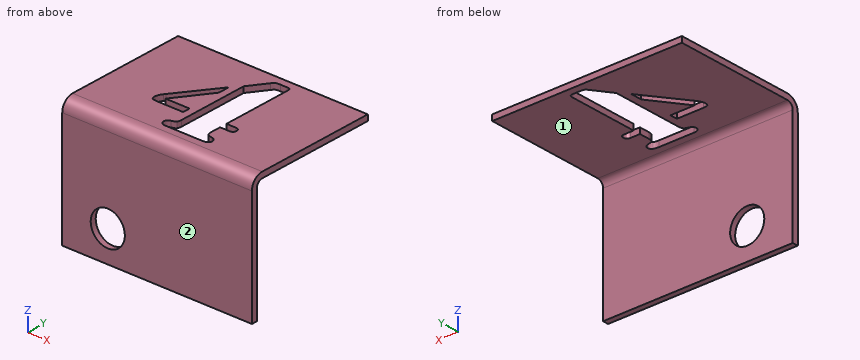
```python
from build123d import *

# Parameters (mm, degrees)
SKETCH1_W            = 50
SKETCH1_H            = 30
BASE_FLANGE1_DEPTH   = 1.51892
EDGE_FLANGE1_DEPTH   = 50
M8_CLEARANCE_HOLE1_D = 9
CUT_EXTRUDE1_DEPTH   = 55.277389816


# Sheet-metal steps are written as plain solids
with BuildPart() as part:
    # Sketch1 → Base-Flange1 (new body)
    with BuildSketch(Plane(origin=(0, 0, 0), x_dir=(1, 0, 0), z_dir=(0, 1, 0))):
        with Locations((0, 15)):
            Rectangle(SKETCH1_W, SKETCH1_H)
    extrude(amount=BASE_FLANGE1_DEPTH)

    # Edge-Flange1 section (across the edge) → Edge-Flange1 (add)
    with BuildSketch(Plane(origin=(-25, 1.51892, 1.5875), x_dir=(0, 0, -1), z_dir=(1, 0, 0))):
        with BuildLine():
            Line((-1.51892, 1.5875), (-1.51892, 33.48108))
            Line((-1.51892, 33.48108), (0, 33.48108))
            Line((0, 33.48108), (0, 1.5875))
            ThreePointArc((0, 1.5875), (0.464967985, 0.464967985), (1.5875, 0))
            Line((1.5875, 0), (1.5875, -1.51892))
            ThreePointArc((1.5875, -1.51892), (-0.609070647, -0.609070647), (-1.51892, 1.5875))
        make_face()
    extrude(amount=EDGE_FLANGE1_DEPTH)

    # M8 Clearance Hole1 (through all)
    with Locations(Plane(origin=(0, 1.51892, 0), x_dir=(1, 0, 0), z_dir=(0, 1, 0))):
        with Locations((-13, 21.89358)):
            Hole(M8_CLEARANCE_HOLE1_D / 2)

    # Sketch11 → Cut-Extrude1 (cut, through all)
    with BuildSketch(Plane.XY.offset(3.10642)):
        with BuildLine():
            Line((-1.313983013, 27.652777778), (1.882197542, 32.167534722))
            add(Edge.make_bspline(
                [(1.882197542, 32.167534722), (1.942990154, 32.25422683), (2.055720733, 32.414984053), (2.238806296, 32.612748461), (2.402031604, 32.768107394), (2.575292151, 32.867707043), (2.775618459, 32.931720261), (3.025586613, 32.967610097), (3.337632557, 33.001581085), (3.567244353, 33.000559396), (3.692961431, 33)],
                knots=[0, 0, 0, 0, 1.195193305, 2.216302741, 3.043406804, 3.730660832, 4.454688059, 5.406997193, 6.580278791, 8, 8, 8, 8], degree=3))
            Line((3.692961431, 33), (5.467266987, 33))
            add(Edge.make_bspline(
                [(5.467266987, 33), (5.577064754, 32.996788141), (5.77366231, 32.991037172), (6.032013828, 32.946349792), (6.233785133, 32.868906911), (6.308685128, 32.770626919), (6.342266987, 32.7265625)],
                knots=[0, 0, 0, 0, 1.37922202, 2.469555487, 3.31381609, 4, 4, 4, 4], degree=3))
            add(Edge.make_bspline(
                [(6.342266987, 32.7265625), (6.362353673, 32.676444121), (6.407796446, 32.563059661), (6.435754197, 32.362580464), (6.463680714, 32.121762999), (6.46375452, 31.94690658), (6.463794764, 31.8515625)],
                knots=[0, 0, 0, 0, 0.726336959, 1.64321602, 2.714914776, 4, 4, 4, 4], degree=3))
            Line((6.463794764, 31.8515625), (6.463794764, 13.555555556))
            Line((6.463794764, 13.555555556), (9.028030875, 13.555555556))
            add(Edge.make_bspline(
                [(9.028030875, 13.555555556), (9.165896219, 13.546190847), (9.419639988, 13.528954925), (9.754751832, 13.344043), (9.938206738, 13.006772556), (9.954683864, 12.75366768), (9.963794764, 12.613715278)],
                knots=[0, 0, 0, 0, 1.088306732, 2.003049094, 2.895801301, 4, 4, 4, 4], degree=3))
            add(Edge.make_bspline(
                [(9.963794764, 12.613715278), (9.953871828, 12.46514926), (9.935630574, 12.192041557), (9.724439936, 11.830921806), (9.34752556, 11.633510395), (9.062693451, 11.619043932), (8.906503098, 11.611111111)],
                knots=[0, 0, 0, 0, 1.064523988, 1.9569058, 2.879650172, 4, 4, 4, 4], degree=3))
            Line((8.906503098, 11.611111111), (6.463794764, 11.611111111))
            Line((6.463794764, 11.611111111), (6.463794764, 8.955729167))
            add(Edge.make_bspline(
                [(6.463794764, 8.955729167), (6.465256175, 8.831576902), (6.468012829, 8.59738883), (6.54117183, 8.277019076), (6.627610008, 7.995757008), (6.738971671, 7.851550593), (6.791919764, 7.782986111)],
                knots=[0, 0, 0, 0, 1.194828702, 2.253802076, 3.169751524, 4, 4, 4, 4], degree=3))
            add(Edge.make_bspline(
                [(6.791919764, 7.782986111), (6.846531378, 7.730010442), (6.944813868, 7.634672101), (7.100203776, 7.539617352), (7.27176022, 7.495886787), (7.482006075, 7.440754455), (7.780922877, 7.369916119), (8.00732939, 7.311522722), (8.134801709, 7.278645833)],
                knots=[0, 0, 0, 0, 0.938335918, 1.688688255, 2.210658911, 3.11404715, 4.375139053, 6, 6, 6, 6], degree=3))
            add(Edge.make_bspline(
                [(8.134801709, 7.278645833), (8.292748806, 7.235768373), (8.582838073, 7.157018646), (8.93848225, 6.903617509), (9.154259726, 6.543911357), (9.175060001, 6.272945389), (9.186016987, 6.130208333)],
                knots=[0, 0, 0, 0, 1.146809638, 2.106256929, 3.002430776, 4, 4, 4, 4], degree=3))
            add(Edge.make_bspline(
                [(9.186016987, 6.130208333), (9.17899553, 6.042021554), (9.165241661, 5.869278259), (9.05359535, 5.623704764), (8.862916658, 5.414842755), (8.700602579, 5.306421387), (8.614836431, 5.249131944)],
                knots=[0, 0, 0, 0, 0.958462782, 1.877469862, 2.878463071, 4, 4, 4, 4], degree=3))
            add(Edge.make_bspline(
                [(8.614836431, 5.249131944), (8.534946889, 5.209690912), (8.357433658, 5.122053596), (8.034892473, 5.049887402), (7.643647807, 5.011727038), (7.359176572, 5.004119856), (7.205114209, 5)],
                knots=[0, 0, 0, 0, 0.737495844, 1.638703467, 2.721182046, 4, 4, 4, 4], degree=3))
            Line((7.205114209, 5), (6.482023931, 5))
            Line((6.482023931, 5), (-1.33221218, 5))
            Line((-1.33221218, 5), (-1.958080236, 5))
            add(Edge.make_bspline(
                [(-1.958080236, 5), (-2.089881071, 5.00416961), (-2.333985762, 5.01189203), (-2.66895246, 5.049646344), (-2.944215562, 5.122135251), (-3.089638978, 5.209698692), (-3.155128847, 5.249131944)],
                knots=[0, 0, 0, 0, 1.275972689, 2.363193818, 3.262881972, 4, 4, 4, 4], degree=3))
            add(Edge.make_bspline(
                [(-3.155128847, 5.249131944), (-3.228690112, 5.307025561), (-3.370553227, 5.418673569), (-3.534127754, 5.628370393), (-3.631583422, 5.871216423), (-3.641971775, 6.042227184), (-3.647316347, 6.130208333)],
                knots=[0, 0, 0, 0, 1.065580224, 2.054974559, 2.999328622, 4, 4, 4, 4], degree=3))
            add(Edge.make_bspline(
                [(-3.647316347, 6.130208333), (-3.640263565, 6.272706576), (-3.626998251, 6.540726201), (-3.433693624, 6.890936561), (-3.132521052, 7.155953313), (-2.874583156, 7.235736523), (-2.735858013, 7.278645833)],
                knots=[0, 0, 0, 0, 1.059227515, 1.99226149, 2.920190418, 4, 4, 4, 4], degree=3))
            add(Edge.make_bspline(
                [(-2.735858013, 7.278645833), (-2.628596603, 7.311344749), (-2.438567719, 7.36927554), (-2.186761633, 7.442084104), (-2.007968702, 7.494958163), (-1.85808029, 7.542989269), (-1.717703343, 7.629665553), (-1.64102438, 7.729186896), (-1.599573291, 7.782986111)],
                knots=[0, 0, 0, 0, 1.58908833, 2.815296579, 3.714312333, 4.231769587, 5.044130571, 6, 6, 6, 6], degree=3))
            add(Edge.make_bspline(
                [(-1.599573291, 7.782986111), (-1.553206662, 7.852049956), (-1.454388083, 7.999241828), (-1.378985552, 8.277685094), (-1.321790362, 8.598779226), (-1.316693685, 8.831797968), (-1.313983013, 8.955729167)],
                knots=[0, 0, 0, 0, 0.808960821, 1.724092502, 2.789556825, 4, 4, 4, 4], degree=3))
            Line((-1.313983013, 8.955729167), (-1.313983013, 27.652777778))
        make_face()
        with BuildLine():
            Line((-3.258427458, 25.404513889), (-3.258427458, 22.408854167))
            Line((-3.258427458, 22.408854167), (-9.608253847, 13.555555556))
            Line((-9.608253847, 13.555555556), (-3.258427458, 13.555555556))
            Line((-3.258427458, 13.555555556), (-3.258427458, 11.611111111))
            Line((-3.258427458, 11.611111111), (-10.319191347, 11.611111111))
            add(Edge.make_bspline(
                [(-10.319191347, 11.611111111), (-10.453058826, 11.614326043), (-10.697535464, 11.62019734), (-11.030466888, 11.667544917), (-11.298322213, 11.741534104), (-11.508093604, 11.857572638), (-11.651421931, 12.033101366), (-11.747915639, 12.255162092), (-11.806947017, 12.529695798), (-11.811530061, 12.730869026), (-11.813983013, 12.838541667)],
                knots=[0, 0, 0, 0, 1.411258846, 2.577323645, 3.536890269, 4.331839585, 5.059357258, 5.881395614, 6.866073128, 8, 8, 8, 8], degree=3))
            add(Edge.make_bspline(
                [(-11.813983013, 12.838541667), (-11.805252819, 12.985215395), (-11.787239389, 13.287854337), (-11.650289436, 13.74422143), (-11.429079802, 14.206722525), (-11.230633277, 14.501805138), (-11.127351069, 14.655381944)],
                knots=[0, 0, 0, 0, 0.891359058, 1.839183926, 2.875395504, 4, 4, 4, 4], degree=3))
            Line((-11.127351069, 14.655381944), (-10.823531625, 15.080729167))
            Line((-10.823531625, 15.080729167), (-3.258427458, 25.404513889))
        make_face()
    extrude(amount=-CUT_EXTRUDE1_DEPTH, mode=Mode.SUBTRACT)


solid = part.part
```
Input: part model. Units: mm. Frame: model coordinates. Face numbers are marked on the shaded views. A direction names the side the tool comes from. Give positions to 0.01 mm unless a question says otherwise; leave off trailing zeros. Order: outer loops, then holes, each group sorted by start corner. A loop starts at its lowest first (then second) coordinate and runs counter-clockwise, first axis right, second up. Notation, with made-up numbers: M 32,-7.75 L 44,-7.75 A19 ccw 44,1.25 Z; hole C 0,74 d8. An arc over 180 degrees is marked long. Return JSON: item names as keys, results as strings.
1) Section query D-D on x = 12.5. Output: boundary loops of the cut face in (y, z) (1 decimal).
Taken from the geometry:
{"outline": "M 0,-30 L 1.5,-30 L 1.5,0 A1.6 cw 3.1,1.6 L 35,1.6 L 35,3.1 L 3.1,3.1 A3.1 ccw 0,0 Z"}
2) Section query B-B on y = 26. Output: boundary loops of the cut face in (x, z), and give its area (3 significant figures).
Taken from the geometry:
{"outline": "M -25,1.59 L -1.31,1.59 L -1.31,3.11 L -25,3.11 Z; M 6.46,1.59 L 25,1.59 L 25,3.11 L 6.46,3.11 Z", "area": "64.1 mm2"}
3) Line query: L1, parallel to Y at x = 22, z = -17; L2, parallel to Z at x = -13, y = 1.1; L3, parallel to Z at x = -13, y = 0.5. Output: solid intervals per line, ascending. Write a range as [from, to].
Taken from the geometry:
{"L1": "y = [0, 1.52]", "L2": "z = [-30, -26.39], [-17.39, 2.37]", "L3": "z = [-30, -26.39], [-17.39, 1.69]"}
4) Contact query for flat-ended pins moving along their axis: pin 1 (8 mm diameter, centred on x = -12, z = -9, fed in from +Y); pin 2 (6 mm diameter, centred on x = -13, y = 22.5, fed in from -Z); pin 3 (8 mm diameter, centred on x = -13, z = -21.89, fed in from +Y); pin 4 (1.7 mm diameter, centred on x = 4.5, z = 2.5, fed in from -Y). Output: stop coordinate, or through.
Taken from the geometry:
{"pin 1": "stops at y = 1.52", "pin 2": "stops at z = 1.59", "pin 3": "passes through", "pin 4": "stops at y = 0.47"}
5) Section query A-A on x = -13. Output: boundary loops of the cut face in (y, z) (1 decimal).
Taken from the geometry:
{"outline": "M 0,-30 L 1.5,-30 L 1.5,-26.4 L 0,-26.4 Z; M 0,-17.4 L 1.5,-17.4 L 1.5,0 A1.6 cw 3.1,1.6 L 35,1.6 L 35,3.1 L 3.1,3.1 A3.1 ccw 0,0 Z"}
6) Access query for the marked faces 1 and 2. Directions: +Z, -Z, +X, -X, +Y, -Y. A direction counts if a zero-diameter tool reaches every point of the face in a straight line with its end or side. Return the directions, or none.
Taken from the geometry:
{"face 1": "-Z, +X, -X, +Y", "face 2": "+Z, -Z, +X, -X, -Y"}
7) Section query C-C on y = 21.5. Output: boundary loops of the cut face in (x, z), and give its area (3 significant figures).
Taken from the geometry:
{"outline": "M -25,1.59 L -6.12,1.59 L -6.12,3.11 L -25,3.11 Z; M -3.91,1.59 L -1.31,1.59 L -1.31,3.11 L -3.91,3.11 Z; M 6.46,1.59 L 25,1.59 L 25,3.11 L 6.46,3.11 Z", "area": "60.8 mm2"}
